Can you work these out from the model? Positions are in its coordinate system, mm. Face numbers are marked on the shaded views. A direction names the side the tool comes from. Coordinates: 2 decimals unless noted, no trailing zeros. Loops run counter-clockwise (first coordinate to the right, second up) from the corner with the lowest first, then second, coordinate; pieces in that order, holes last.
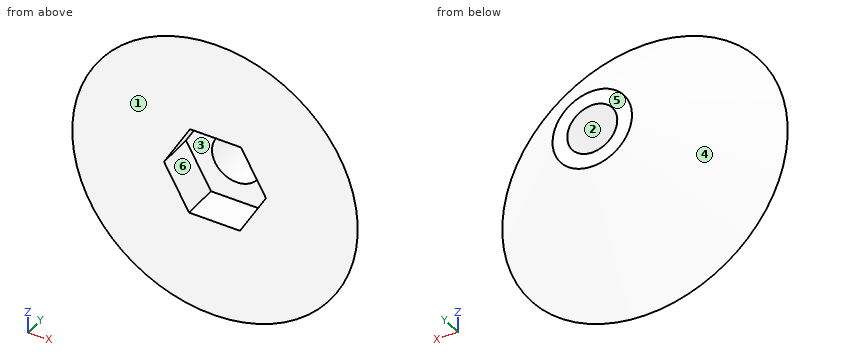
```python
from build123d import *

# Parameters (mm, degrees)
CUT_EXTRUDE1_DEPTH = 2.5


with BuildPart() as part:
    # Sketch1 → Revolve1 (revolve)
    with BuildSketch(Plane.XY, mode=Mode.PRIVATE) as revolve1_sk:
        Polygon((-2.7, 6), (-9.7, 0), (-1.7, 0), (-1.7, 6), align=None)
    revolve(revolve1_sk.sketch.rotate(Axis((0, 11.326530612, 0), (0, -1, 0)), 270), axis=Axis((0, 11.326530612, 0), (0, -1, 0)))

    # Sketch2 → Cut-Extrude1 (cut)
    with BuildSketch(Plane.XZ):
        Polygon((1.697539741, -3.019662039), (3.463873907, -0.03971848), (1.766334166, 2.979943559), (-1.697539741, 3.019662039), (-3.463873907, 0.03971848), (-1.766334166, -2.979943559), align=None)
    extrude(amount=-CUT_EXTRUDE1_DEPTH, mode=Mode.SUBTRACT)


solid = part.part
```
(1) Which directions (+Z, -Z, +X, -X, +Y, -Y) give clear straight access to the entire face, cutting with the end or side of a thin tool? Please do the marked faces 5 and 6.
Check values:
face 5: +Z, -Z, +X, -X, +Y
face 6: -Y
(2) If we mould it in two halves opening along X, with no side actions, what happens to the marked faces 1, 2, 3 and 4? For each: released by +X, released by -X, zero draft, split by the parting line, or undercut.
Check values:
face 1: zero draft
face 2: undercut
face 3: undercut
face 4: split by the parting line
(3) I want a section at B-B on x = 0. Write out the boundary of the cut face in (y, z), then the cut area to 3 significant figures.
Check values:
outline: (0, -9.7) - (6, -2.7) - (6, -1.7) - (2.5, -1.7) - (2.5, -3) - (0, -3) - close; (0, 3) - (2.5, 3) - (2.5, 1.7) - (6, 1.7) - (6, 2.7) - (0, 9.7) - close
area: 47.5 mm2
(4) I want a section at A-A on y = 0.55. Write out the boundary of the cut face in (x, z).
Check values:
outline: circle Ø18.12 at (0, 0); hole (-3.46, 0.04) - (-1.77, -2.98) - (1.7, -3.02) - (3.46, -0.04) - (1.77, 2.98) - (-1.7, 3.02) - close
(5) If I drill on probe 1 along X at (y, z) = (5.1, 0); probe 2 along X at (y, z) = (3.85, 0); probe 3 along Y at (x, z) = (5.75, -7.5), over which ranges is the centre line in solid material (lowest first)?
Check values:
probe 1: x = -3.75 to -1.7, 1.7 to 3.75
probe 2: x = -5.21 to -1.7, 1.7 to 5.21
probe 3: y = 0 to 0.21
(6) I'm going to push flat-ended pins straight in: pin 1 (4 mm diameter, centred on x = -0.5, z = 4, fed in from +Y); pin 2 (6 mm diameter, centred on x = -7, z = 2, fed in from +Y); pin 3 (1 mm diameter, centred on y = 2.5, z = 6, fed in from +X); pin 4 (4 mm diameter, centred on x = -7, z = 5, fed in from +Y). Where does each tip first touch, or does it pass through?
Check values:
pin 1: stops at y = 6
pin 2: stops at y = 4.65
pin 3: stops at x = 4.48
pin 4: stops at y = 2.66
(7) I want a section at C-C on y = 4.7. Write out the boundary of the cut face in (x, z).
Check values:
outline: circle Ø8.43 at (0, 0); hole circle Ø3.4 at (0, 0)
